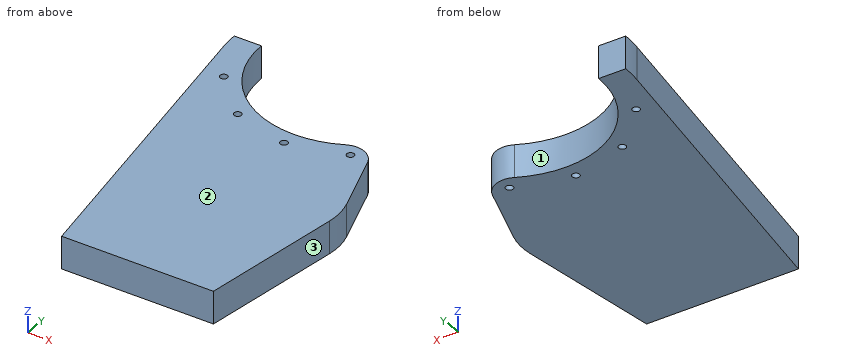
from build123d import *

# Parameters (mm, degrees)
SKETCH1_R           = 1.7
BOSS_EXTRUDE1_DEPTH = 15
FILLET1_R           = 10
FILLET2_R           = 30


with BuildPart() as part:
    # Sketch1 → Boss-Extrude1 (new body)
    with BuildSketch(Plane.XY):
        with BuildLine():
            Line((-57.5, 0), (-45, 0))
            ThreePointArc((-45, 0), (-18.212102581, -41.149961356), (30.258636425, -33.307880775))
            Line((30.258636425, -33.307880775), (46.0437747, -81.254716073))
            Line((46.0437747, -81.254716073), (35.213577586, -154.047675233))
            Line((35.213577586, -154.047675233), (-34.786422414, -154.047675233))
            Line((-34.786422414, -154.047675233), (-56.849444808, -8.625))
            ThreePointArc((-56.849444808, -8.625), (-57.337130537, -4.324749908), (-57.5, 0))
        make_face()
        with Locations((0, -52)):
            Circle(SKETCH1_R, mode=Mode.SUBTRACT)
        with Locations((-26, -45.033320997)):
            Circle(SKETCH1_R, mode=Mode.SUBTRACT)
        with Locations((-45.033320997, -26)):
            Circle(SKETCH1_R, mode=Mode.SUBTRACT)
        with Locations((26, -45.033320997)):
            Circle(SKETCH1_R, mode=Mode.SUBTRACT)
    extrude(amount=BOSS_EXTRUDE1_DEPTH)

    # Fillet1
    fillet1_edges = [part.edges().sort_by_distance(p)[0] for p in [
        (30.258636425, -33.307880775, 7.5),
    ]]
    fillet(fillet1_edges, radius=FILLET1_R)

    # Fillet2
    fillet2_edges = [part.edges().sort_by_distance(p)[0] for p in [
        (46.0437747, -81.254716073, 7.5),
    ]]
    fillet(fillet2_edges, radius=FILLET2_R)


solid = part.part
The listing builds one solid part. Answer for the finished solid, in the listing's coordinates (mm). Face numbers are marked on the shaded views. Coordinates: 2 decimals unless noted, no trailing zeros. Loops run counter-clockwise (first coordinate to the right, second up) from the corner with the lowest first, then second, coordinate; pieces in that order, holes last. Notation, with made-up numbers: (16, -39.5) -> (74, -39.5) arc R23 ccw to (74, -20.5) -> close; hole circle Ø5 at (67.5, -0.75). An arc over 180 degrees is marked (long way). Write item = value, one per line. Start each with the question number.
1) A cutting plane is placed at A-A (x = 0). Give the vertices of the cut face in (y, z).
2) Given pin 1 Ø1 at (x, z) = (13.5, 5.5) entering from +Y; pin 2 Ø5 at (x, y) = (17, -69.5) entering from -Z; pin 3 Ø1.5 at (y, z) = (-26, 13) entering from +X; pin 4 Ø1.5 at (x, z) = (12.5, 4) entering from +Y, each flat-ended and moving along its own axis, determine where each tip first touches the part or whether it passes through.
3) Straight lines are drawn through the part: line 1 (X direction, y = -40, z = 9.75); line 2 (Y direction, x = -12, z = 11.5); line 3 (Y direction, x = 26, z = 11.75). For each, find the intervals that lie inside material, in ascending order. Write a range as from..to.
4) A cutting plane is placed at B-B (y = -52). Give the vertices of the cut face in (x, z), then the cut area to 3 significant figures.
5) A cutting plane is placed at D-D (x = -38.5). Give the vertices of the cut face in (y, z).
6) A cutting plane is placed at C-C (z = 4.5). Give the vertices of the cut face in (x, y) (3 decimals), then the cut area to 3 significant figures.
7) The mould has two halves that part along X. Classify the marked faces 1, 2 and 3: released by +X, released by -X, zero draft, split by the parting line, or undercut.
Responses:
q1.outline = (-154.05, 0) -> (-53.7, 0) -> (-53.7, 15) -> (-154.05, 15) -> close; (-50.3, 0) -> (-45, 0) -> (-45, 15) -> (-50.3, 15) -> close
q2.pin_1 = -42.77
q2.pin_2 = 0
q2.pin_3 = -36.19
q2.pin_4 = -43.01
q3.line_1 = -52.09..-20.62, 20.63..29.19
q3.line_2 = -154.05..-43.37
q3.line_3 = -154.05..-46.73, -43.33..-39.1
q4.outline = (-50.27, 0) -> (-1.7, 0) -> (-1.7, 15) -> (-50.27, 15) -> close; (1.7, 0) -> (36.41, 0) -> (36.41, 15) -> (1.7, 15) -> close
q4.area = 1,250 mm²
q5.outline = (-129.57, 0) -> (-23.3, 0) -> (-23.3, 15) -> (-129.57, 15) -> close
q6.outline = (-57.5, 0) arc R57.5 ccw to (-56.849, -8.625) -> (-34.786, -154.048) -> (35.214, -154.048) -> (44.997, -88.292) arc R30 ccw to (43.819, -74.496) -> (34.407, -45.909) arc R10 ccw to (20.38, -40.121) arc R45 cw to (-45, 0) -> close; hole circle Ø3.4 at (-45.033, -26); hole circle Ø3.4 at (-26, -45.033); hole circle Ø3.4 at (0, -52); hole circle Ø3.4 at (26, -45.033)
q6.area = 10,000 mm²
q7.face_1 = undercut
q7.face_2 = zero draft
q7.face_3 = released by +X
